Autodesk Inventor part; units mm, degrees
ref_plane "YZ Plane" through (0, 0, 0) normal (1, 0, 0) x (0, 1, 0)
ref_plane "XZ Plane" through (0, 0, 0) normal (0, 1, 0) x (-1, 0, 0)
ref_plane "XY Plane" through (0, 0, 0) normal (0, 0, 1) x (1, 0, 0)
sketch "Sketch1" plane through (0, 0, 0) normal (0, 1, 0) x (-1, 0, 0)
  arc A0 (334.15, 5.5) -> (337.85, 5.5) centre (336, 5.5) ccw
  arc A1 (345.85, 13.5) -> (342.15, 13.5) centre (344, 13.5) ccw
  arc A2 (329.85, 13.5) -> (326.15, 13.5) centre (328, 13.5) ccw
  arc A3 (328.4931, 19.1569) -> (332.1931, 19.1569) centre (330.3431, 19.1569) ccw
  arc A4 (334.15, 21.5) -> (337.85, 21.5) centre (336, 21.5) ccw
  arc A5 (332, 13.5) -> (340, 13.5) centre (336, 13.5) ccw
  arc A6 (337.85, 181.5) -> (334.15, 181.5) centre (336, 181.5) ccw
  arc A7 (334.15, 197.5) -> (337.85, 197.5) centre (336, 197.5) ccw
  arc A8 (340, 189.5) -> (332, 189.5) centre (336, 189.5) ccw
  arc A9 (329.85, 189.5) -> (326.15, 189.5) centre (328, 189.5) ccw
  arc A10 (345.85, 189.5) -> (342.15, 189.5) centre (344, 189.5) ccw
  line L0 (352, 176) -> (352, 203)
  arc A11 (244, 13.5) -> (236, 13.5) centre (240, 13.5) ccw
  arc A12 (241.85, 21.5) -> (238.15, 21.5) centre (240, 21.5) ccw
  arc A13 (244, 189.5) -> (236, 189.5) centre (240, 189.5) ccw
  arc A14 (233.85, 189.5) -> (230.15, 189.5) centre (232, 189.5) ccw
  line L1 (228.8458, 84.7173) -> (228.8458, 88.629)
  arc A15 (336, 137.5) -> (336, 145.5) centre (336, 141.5) ccw
  arc A16 (336, 121.5) -> (336, 129.5) centre (336, 125.5) ccw
  arc A17 (336, 105.5) -> (336, 113.5) centre (336, 109.5) ccw
  arc A18 (336, 89.5) -> (336, 97.5) centre (336, 93.5) ccw
  arc A19 (336, 73.5) -> (336, 81.5) centre (336, 77.5) ccw
  arc A20 (336, 57.5) -> (336, 65.5) centre (336, 61.5) ccw
  arc A21 (336, 41.5) -> (336, 49.5) centre (336, 45.5) ccw
  arc A22 (336, 25.5) -> (336, 33.5) centre (336, 29.5) ccw
  arc A23 (336, 153.5) -> (336, 161.5) centre (336, 157.5) ccw
  arc A24 (336, 169.5) -> (336, 177.5) centre (336, 173.5) ccw
  arc A25 (260, 189.5) -> (252, 189.5) centre (256, 189.5) ccw
  arc A26 (276, 189.5) -> (268, 189.5) centre (272, 189.5) ccw
  arc A27 (292, 189.5) -> (284, 189.5) centre (288, 189.5) ccw
  arc A28 (308, 189.5) -> (300, 189.5) centre (304, 189.5) ccw
  arc A29 (324, 189.5) -> (316, 189.5) centre (320, 189.5) ccw
  line L2 (352, 203) -> (228.8458, 203)
  line L3 (228.8458, 203) -> (228.8458, 0)
  line L4 (228.8458, 0) -> (352, 0)
  line L5 (352, 0) -> (352, 203)
  line L6 (-2.54, -2.54) -> (116.84, -2.54)
  line L7 (116.84, -2.54) -> (116.84, 193.04)
  line L8 (116.84, 193.04) -> (-2.54, 193.04)
  line L9 (-2.54, 193.04) -> (-2.54, -2.54)
  line L10 (-2.54, 95.25) -> (-2.54, 183.2483)
  line L11 (-2.54, 183.2483) -> (116.84, 183.2483)
  line L12 (-2.54, 183.2483) -> (-2.54, 7.2517)
  line L13 (-2.54, 7.2517) -> (116.84, 7.2517)
  line L14 (116.84, 183.2483) -> (100.838, 183.2483)
  line L15 (100.838, 183.2483) -> (100.838, 7.2517)
  circle A30 centre (100.838, 183.2483) radius 4.0005
  circle A31 centre (84.836, 183.2483) radius 4.0005
  circle A32 centre (68.834, 183.2483) radius 4.0005
  circle A33 centre (52.832, 183.2483) radius 4.0005
  circle A34 centre (36.83, 183.2483) radius 4.0005
  circle A35 centre (20.828, 183.2483) radius 4.0005
  circle A36 centre (4.826, 183.2483) radius 4.0005
  line L16 (100.838, 183.2483) -> (100.838, 175.2473)
  circle A37 centre (100.838, 175.2473) radius 1.8542
  line L17 (100.838, 183.2483) -> (104.5464, 183.2483)
  line L18 (100.838, 183.2483) -> (108.839, 183.2483)
  circle A38 centre (108.839, 183.2483) radius 1.8542
  point P0 (287.9997, 29.5)
  point P1 (228.8458, 85.5356)
  dimension "d0" = 203
  dimension "d1" = 123.1542
  dimension "d2" = 119.38
  dimension "d3" = 195.58
  dimension "d4" = 87.9983
  dimension "d5" = 175.9966
  dimension "d6" = 16.002
  dimension "d7" = 8.001
  dimension "d10" = 16.002
  dimension "d15" = 8.001
  dimension "d16" = 3.7084
  dimension "d17" = 3.7084
  dimension "d18" = 8.001
  dimension "d19" = 3.7084
extrude "Extrusion1" add sketch "Sketch1" along normal blind 3.175 contours L9 L13 L7 L6 | L9 L11 A36 A35 A34 A33 A32 A31 A30 L15 A37 L13 | L13 L15 A37 A30 L11 A38 L7 | L11 A38 A30 A31 A32 A33 A34 A35 A36 L9 L8 L7 | A37 L15 | L15 A37 | A38 L11 | L11 A38 | A36 L11 | L11 A36 | A30 L11 L15 | L15 L11 A30 | L11 A30 | A35 L11 | L11 A35 | A31 L11 | L11 A31 | A34 L11 | L11 A34 | A32 L11 | L11 A32 | A33 L11 | L11 A33
extrude "Extrusion2" cut sketch "Sketch1" along normal blind 3.175 contours A37 L15 | L15 A37 | A38 L11 | L11 A38
pattern_linear "Rectangular Pattern1" count 7 spacing 16.002 along (1, 0, 0) of "Extrusion2"
pattern_linear "Rectangular Pattern2" count 12 spacing 16.002 along (0, 0, -1) of "Extrusion2"
sketch "Sketch2" plane through (0, 3.175, 0) normal (0, 1, 0) x (1, 0, 0)
  arc A0 (-101.4053, 2.54) -> (-100.2707, 2.54) centre (-100.838, 0.7747) ccw
  line L0 (2.54, 2.54) -> (-100.2707, 2.54)
  line L1 (-101.4053, 2.54) -> (-100.2707, 2.54)
  point P0 (0, 0)
extrude "Extrusion3" add sketch "Sketch2" against normal up to surface (3.175 mm away)
sketch "Sketch3" plane through (0, 3.175, 0) normal (0, 1, 0) x (1, 0, 0)
  line L0 (2.54, 2.54) -> (-116.84, 2.54)
  circle A0 centre (-108.839, -7.2263) radius 1.8542
  circle A1 centre (-100.838, -15.2273) radius 1.8542
  circle A2 centre (-108.839, -7.2263) radius 1.8542
  circle A3 centre (-100.838, -15.2273) radius 1.8542
  circle A4 centre (-92.837, -7.2263) radius 1.8542
  circle A5 centre (-84.836, -15.2273) radius 1.8542
  circle A6 centre (-76.835, -7.2263) radius 1.8542
  circle A7 centre (-68.834, -15.2273) radius 1.8542
  circle A8 centre (-60.833, -7.2263) radius 1.8542
  circle A9 centre (-52.832, -15.2273) radius 1.8542
  circle A10 centre (-44.831, -7.2263) radius 1.8542
  circle A11 centre (-36.83, -15.2273) radius 1.8542
  circle A12 centre (-28.829, -7.2263) radius 1.8542
  circle A13 centre (-20.828, -15.2273) radius 1.8542
  circle A14 centre (-12.827, -7.2263) radius 1.8542
  circle A15 centre (-4.826, -15.2273) radius 1.8542
  point P0 (0, 0)
  dimension "d34" = 16.002
extrude "Extrusion4" cut sketch "Sketch3" against normal blind 3.175 contours A4 | A5 | A6 | A7 | A8 | A9 | A10 | A11 | A12 | A13 | A14 | A15
sketch "Sketch4" plane through (0, 3.175, 0) normal (0, 1, 0) x (1, 0, 0)
  circle A0 centre (-36.83, -15.2273) radius 1.8542
  circle A1 centre (-52.832, -15.2273) radius 1.8542
  circle A2 centre (-68.834, -15.2273) radius 1.8542
  line L0 (2.54, -193.04) -> (2.54, 2.54)
  circle A3 centre (-36.83, -175.2473) radius 1.8542
  circle A4 centre (-52.832, -175.2473) radius 1.8542
  circle A5 centre (-68.834, -175.2473) radius 1.8542
  line L1 (-68.834, -175.2473) -> (-68.834, -15.2273)
  line L2 (-68.834, -15.2273) -> (-52.832, -15.2273)
  line L3 (-52.832, -15.2273) -> (-52.832, -175.2473)
  line L4 (-52.832, -175.2473) -> (-36.83, -175.2473)
  line L5 (-36.83, -175.2473) -> (-36.83, -15.2273)
  circle A6 centre (-68.834, -95.2373) radius 1.8542
  circle A7 centre (-52.832, -95.2373) radius 1.8542
  circle A8 centre (-36.83, -95.2373) radius 1.8542
  point P0 (0, 0)
  dimension "d41" = 3.7084
  dimension "d42" = 3.7084
  dimension "d43" = 3.7084
extrude "Extrusion5" cut sketch "Sketch4" against normal blind 25.4 contours A6 L1 | L1 A6 | A7 L3 | L3 A7 | A8 L5 | L5 A8
sketch "Sketch5" plane through (0, 3.175, 0) normal (0, 1, 0) x (1, 0, 0)
  circle A0 centre (-4.826, -159.2453) radius 1.8542
  point P0 (0, 0)
  dimension "d46" = 3.7084
extrude "Extrusion6" cut sketch "Sketch5" against normal blind 25.4
pattern_linear "Rectangular Pattern3" count 9 spacing 16.002 along (0, 0, -1) of "Extrusion6"
properties part number "Electronics Board" material "ABS Plastic"
Geometry: final body of the model. Coordinates: model frame, mm. Coordinates: 2 decimals unless noted, no trailing zeros. Order: outer loops, then holes, each group sorted by start corner. A loop starts at its lowest first (then second) coordinate and runs counter-clockwise, first axis right, second up. Notation, with made-up numbers: M 25,15 L 82,15 A22 ccw 82,26 Z; hole C -7,38.5 d7. An arc over 180 degrees is marked long. One line per question, with ' | ' between items. Start each with the question number.
Item 1: Cut plane A-A, the plane x = -36.83. Return the cut outline in (y, z) (1 decimal), then the cut area to 3 significant figures.
Item 2: Cut plane B-B, the plane y = 0.6. Count the separate pieces of the cut face and the enclosed holes in it, then the cut area to 3 significant figures.
Item 3: Ray query, probe 1 along Z at (x, y) = (-12.5, 0.95); probe 2 along Z at (x, y) = (-93.5, 0.6); probe 3 along X at (y, z) = (2.4, 135). Return the intervals inside material, ascending. Write a range as [from, to].
Item 4: Pin query (flat end, axial travel): pin 1 Ø2 at (x, z) = (-4.83, 15.23) entering from +Y. Return the tip coordinate at first contact, or that it passes through.
A:
1) outline: M 0,-2.5 L 3.2,-2.5 L 3.2,13.4 L 0,13.4 Z; M 0,17.1 L 3.2,17.1 L 3.2,93.4 L 0,93.4 Z; M 0,97.1 L 3.2,97.1 L 3.2,173.4 L 0,173.4 Z; M 0,177.1 L 3.2,177.1 L 3.2,193 L 0,193 Z | area: 586 mm2
2) separate pieces: 1 | enclosed holes: 59 | area: 22,700 mm2
3) probe 1: z = [-2.54, 5.4], [9.05, 181.42], [185.07, 193.04] | probe 2: z = [-2.54, 5.49], [8.96, 181.52], [184.98, 193.04] | probe 3: x = [-116.84, -110.68], [-107, 2.54]
4) pin 1: passes through
